Design review of the part built by this model. Coordinates are the model's own, in mm. A direction names the side the tool comes from. Coordinates: 2 decimals unless noted, no trailing zeros. Loops run counter-clockwise (first coordinate to the right, second up) from the corner with the lowest first, then second, coordinate; pieces in that order, holes last. Notation, with made-up numbers: (75, 41) -> (134, 41) arc R17 ccw to (134, 61) -> close; hole circle Ø6 at (74, -37). An arc over 180 degrees is marked (long way). Use CSV: the item, a comma, the result in double quotes.
```python
from build123d import *

# Parameters (mm, degrees)
SKETCH2_R           = 1.75
BOSS_EXTRUDE3_DEPTH = 5


with BuildPart() as part:
    # Sketch2 → Boss-Extrude3 (new body)
    with BuildSketch(Plane(origin=(0, 0, 0), x_dir=(1, 0, 0), z_dir=(0, 1, 0))):
        Polygon((-214, -48.75), (-207, -44.75), (-200, -48.75), (-200, -56.75), (-202, -56.75), (-202, -61.75), (-212, -61.75), (-212, -56.75), (-214, -56.75), align=None)
        with Locations((-207, -50)):
            Circle(SKETCH2_R, mode=Mode.SUBTRACT)
    extrude(amount=BOSS_EXTRUDE3_DEPTH)


solid = part.part
```
Item 1: Add section D-D (x = -203.5). Give the boundary of the cut face in (y, z).
Checked values:
outline,"(0, 46.75) -> (5, 46.75) -> (5, 61.75) -> (0, 61.75) -> close"
Item 2: Add section C-C (x = -212.25). Give the boundary of the cut face in (y, z).
Checked values:
outline,"(0, 47.75) -> (5, 47.75) -> (5, 56.75) -> (0, 56.75) -> close"
Item 3: Add section B-B (y = 1.8). Give the boundary of the cut face in (x, z).
Checked values:
outline,"(-214, 48.75) -> (-207, 44.75) -> (-200, 48.75) -> (-200, 56.75) -> (-202, 56.75) -> (-202, 61.75) -> (-212, 61.75) -> (-212, 56.75) -> (-214, 56.75) -> close; hole circle Ø3.5 at (-207, 50)"
Item 4: Draft analysis for pull direction Z (two halves, no side actions). For faces 1 (the face through (-207.38, 2.46, 51.71)), 2 (the face through (-210.55, 2.46, 46.78)), 3 (the face through (-207, 2, 61.75)), state which applies: pulls with the +Z half, pulls with the -Z half, needs draft (parallel to the pull), parting line crosses it, or undercut.
Checked values:
face 1,"undercut"
face 2,"pulls with the -Z half"
face 3,"pulls with the +Z half"
Item 5: To check wall thickness, follow line 1 along X through (y, z) = (2.45, 50); line 2 along Z through (x, y) = (-205.75, 4); line 3 along X through (y, z) = (0.6, 59.5). State the ranges of each line that lie inside material, in increasing order.
Checked values:
line 1,"-214 to -208.75, -205.25 to -200"
line 2,"45.46 to 48.78, 51.22 to 61.75"
line 3,"-212 to -202"
Item 6: Machinability: for faces 4 (the face through (-200, 2, 53)), 5 (the face through (-212, 2, 59)), 6 (the face through (-202, 2, 59)), which of the approach directions +Z, -Z, +X, -X, +Y, -Y give a long, thin tool a straight path to every point of the face, cutting with its end or side? Answer none if there is none.
Checked values:
face 4,"+Z, -Z, +X, +Y, -Y"
face 5,"+Z, -X, +Y, -Y"
face 6,"+Z, +X, +Y, -Y"
Item 7: Add section A-A (z = 50). Give the boundary of the cut face in (x, y).
Checked values:
outline,"(-214, 0) -> (-208.75, 0) -> (-208.75, 5) -> (-214, 5) -> close; (-205.25, 0) -> (-200, 0) -> (-200, 5) -> (-205.25, 5) -> close"
